Autodesk Inventor part; units mm, degrees
ref_plane "XZ Plane" through (0, 0, 0) normal (0, 1, 0) x (-1, 0, 0)
ref_plane "XY Plane" through (0, 0, 0) normal (0, 0, 1) x (1, 0, 0)
ref_plane "Work Plane1" through (508, 0, 0) normal (1, 0, 0) x (0, 1, 0)
sketch "Sketch13" plane through (508, 0, 0) normal (1, 0, 0) x (0, 1, 0)
  circle A0 centre (0, 0) radius 12.7
  point P0 (0, 0)
  dimension "d79" = 25.4
sketch3d "3D Sketch1"
  line L0 (508, 0, 0) -> (15.7815, 0, 0)
  arc A0 (15.7815, 0, 0) -> (-11.1592, 0.0018, -11.1592) centre (15.7815, 0.0061, -38.1) ccw
  line L1 (-11.1592, 0.0018, -11.1592) -> (-152.6613, 0.0245, -152.6613)
  arc A1 (-152.6613, 0.0245, -152.6613) -> (-179.6051, -38.0755, -179.6051) centre (-152.6644, -38.0755, -152.6644) ccw
  line L2 (-179.6051, -38.0755, -179.6051) -> (-179.6051, -253.9712, -179.6051)
  dimension "d73" = 508
  dimension "d74" = 135
  dimension "d75" = 254
  dimension "d76" = 254
  dimension "d77" = 38.1
  dimension "d78" = 38.1
sweep "Sweep1" add profiles "Sketch13" path "3D Sketch1"
sketch "Sketch14" plane through (-179.6051, -253.9712, -179.6051) normal (0, -1, 0) x (1, 0, 0)
  circle A0 centre (0, 0.1847) radius 15.875
  point P0 (179.6051, 179.6051)
  dimension "d82" = 31.75
extrude "Extrusion1" add sketch "Sketch14" against normal blind 215.9
fillet "Fillet1" radius 3.175 1 edges at (-195.4801, -253.9712, -179.4205)
fillet "Fillet2" radius 1.5875 1 edges at (-195.4801, -38.0712, -179.4205)
equation "\"d78\" = d77"
equation "\"BendRadius\" = Thickness"
equation "\"BendReliefWidth\" = Thickness"
equation "\"BendReliefDepth\" = 0.5 * Thickness"
equation "\"CornerReliefSize\" = 4 * Thickness"
equation "\"MinimumRemnant\" = 2 * Thickness"
equation "\"TransitionRadius\" = BendRadius"
equation "\"JacobiRadiusSize\" = BendRadius"
equation "\"GapSize\" = Thickness"
properties part number "5th Wheel Hitch Part 4"
CAD build for the part. Positions are in the model's coordinates, mm. Give positions to 0.01 mm unless a question says otherwise; leave off trailing zeros. Loops run counter-clockwise (first coordinate to the right, second up) from the corner with the lowest first, then second, coordinate; pieces in that order, holes last. Notation, with made-up numbers: M 53.5,49.25 L 112.5,49.25 A10 cw 112.5,53.25 Z; hole C -25.5,50 d7. An arc over 180 degrees is marked long. One line per question, with ' | ' between items. Start each with the question number.
1. Two-plate mould, pull along Y, no slides. Class faces 1 (the face through (258.45, -2.75, 12.4)), 2 (the face through (-179.7, -38.071, -166.7)), 3 (the face through (-195.465, -146.705, -178.722)): pulls with the +Y half, pulls with the -Y half, needs draft (parallel to the pull), parting line crosses it, or undercut.
2. Saw through at B-B on x = 40. Give the cut face in (y, z).
3. Saw through at A-A on y = -174. Give the cut face in (x, z) (3 decimals).
4. Flat gauge pins, fed straight in: pin 1 (8.5 mm diameter, centred on x = -180, z = -186.5, fed in from +Y); pin 2 (5 mm diameter, centred on x = 146, z = -10, fed in from -Y). Where does each tip first touch, or does it go through?
5. Probe L1, parallel to X at y = -187, z = -180.5; L2, parallel to Y at x = -127, z = -131; L3, parallel to Y at x = -76, z = -79.5. List the from-to ranges inside material, lowest first. Write a range as from..to.
Result sheet:
1) face 1: parting line crosses it | face 2: undercut | face 3: needs draft
2) outline: C 0,0 d25.4
3) outline: C -179.605,-179.42 d31.75
4) pin 1: stops at y = -6.46 | pin 2: stops at y = -10.25
5) L1: x = -195.44..-163.77 | L2: y = -12.36..12.4 | L3: y = -12.44..12.47
